Geometry: final body of the model. Coordinates: model frame, mm. A direction names the side the tool comes from. Coordinates: 2 decimals unless noted, no trailing zeros. Write each loop counter-clockwise with the first axis right and the second up, starting at its lowest first coordinate (ties: lowest second). Pieces come first, ordered by that corner, then holes. Notation, with made-up numbers: (6.25, 43) -> (65.25, 43) arc R4 cw to (65.25, 47) -> close; hole circle Ø8 at (33, -2). An arc over 180 degrees is marked (long way). One line per item, written item: value.
```python
from build123d import *

# Parameters (mm, degrees)
BOSS_EXTRUDE1_DEPTH     = 1.5
CUT_EXTRUDE1_DEPTH      = 41.754559874
CUT_EXTRUDE1_DEPTH_BACK = 41.754559874
SKETCH6_R               = 0.5


with BuildPart() as part:
    # Sketch1 → Revolve1 (revolve)
    with BuildSketch(Plane(origin=(-14.777648988, 30.214835565, 34.561537757), x_dir=(-0.025322831104622072, 0, 0.9996793256964189), z_dir=(0.9996793256964189, 0, 0.025322831104622072)), mode=Mode.PRIVATE) as revolve1_sk:
        Polygon((0.538461916, -0.016033073), (-0.794313715, -0.016033073), (-0.794313715, 12.79633963), (-0.794313715, 13.022686392), (0.228391261, 13.022686392), (0.228391261, 12.79633963), (-0.000563715, 12.79633963), (-0.000563715, 11.466008099), (0.538461916, 11.466008099), align=None)
    revolve(revolve1_sk.sketch.rotate(Axis((-14.757534716, 30.388488917, 33.767478758), (0, 1, 0)), 181.451046455), axis=Axis((-14.757534716, 30.388488917, 33.767478758), (0, 1, 0)))

    # Sketch5 → Boss-Extrude1 (add)
    with BuildSketch(Plane(origin=(0, 30.230868638, 0), x_dir=(1, 0, 0), z_dir=(0, 1, 0))):
        Polygon((-14.723785064, -32.435130513), (-14.791284368, -32.435130513), (-14.791284368, -35.099827002), (-14.723785064, -35.099827002), (1.521158766, -35.099827002), (1.521158766, -32.435130513), align=None)
    extrude(amount=BOSS_EXTRUDE1_DEPTH)

    # Sketch6 → Cut-Extrude1 (cut, two sides: drawn at the far end of the back side and taken through both)
    with BuildSketch(Plane.XZ.offset(-30.230868638).offset(-CUT_EXTRUDE1_DEPTH_BACK)):
        with Locations(Location((0.125166735, 33.767478758, 0), (0, 0, 90))):
            Circle(SKETCH6_R)
    extrude(amount=CUT_EXTRUDE1_DEPTH + CUT_EXTRUDE1_DEPTH_BACK, mode=Mode.SUBTRACT)


solid = part.part
```
(1) Pull-direction query (Y, two-part tool) for faces 1 (the flat face through (-15, 30.231, 34)), 2 (the cylindrical face through (-14, 18, 34)), 3 (the flat face through (-7, 31, 32.435)), 4 (the flat face through (-14, 18.749, 33)); classes: released by +Y, released by -Y, zero draft, split by the parting line, or undercut.
Responses:
face 1: released by +Y
face 2: undercut
face 3: zero draft
face 4: undercut
(2) Section C-C (x = -11.5). Return the cut outline in (y, z), then the cut area to 3 significant figures.
Responses:
outline: (30.23, 32.44) -> (31.73, 32.44) -> (31.73, 35.1) -> (30.23, 35.1) -> close
area: 4.00 mm2
(3) Line query: line 1 (Y direction, x = -5.75, z = 34.35); line 2 (X direction, y = 21, z = 32.7); line 3 (X direction, y = 30.75, z = 32.9). Output: solid intervals per line, ascending. Write a range as [from, to].
Responses:
line 1: y = [30.23, 31.73]
line 2: x = [-15.56, -13.96]
line 3: x = [-14.79, 1.52]
(4) Section A-A (z = 33.6). Return the cut outline in (x, y).
Responses:
outline: (-16.08, 18.75) -> (-15.53, 18.75) -> (-15.53, 17.42) -> (-15.77, 17.42) -> (-15.77, 17.19) -> (-13.75, 17.19) -> (-13.75, 17.42) -> (-13.98, 17.42) -> (-13.98, 18.75) -> (-13.44, 18.75) -> (-13.44, 30.23) -> (-0.35, 30.23) -> (-0.35, 31.73) -> (-14.79, 31.73) -> (-14.79, 30.23) -> (-16.08, 30.23) -> close; (0.6, 30.23) -> (1.52, 30.23) -> (1.52, 31.73) -> (0.6, 31.73) -> close
(5) Reachability of faces 5 (the flat face through (-15, 17.192, 34)), 6 (the cylindrical face through (-15.88, 24.57, 33.05)), 7 (the flat face through (-14.791, 31, 34)) from +Z, -Z, +X, -X, +Y, -Y: full face, straight path, thin tool, end or side. Return the list, or none.
Responses:
face 5: +Z, -Z, +X, -X, -Y
face 6: -Y
face 7: +Z, -Z, -X, +Y
(6) Section D-D (y = 23). Return the cut outline in (x, z).
Responses:
outline: circle Ø2.67 at (-14.76, 33.77)
(7) Section B-B (y = 30.75). Return the cut outline in (x, z).
Responses:
outline: (-14.79, 32.44) -> (1.52, 32.44) -> (1.52, 35.1) -> (-14.79, 35.1) -> close; hole circle Ø1 at (0.13, 33.77)
(8) First-contact query: pin 1 (1.5 mm diameter, centred on y = 30, z = 34, fed in from -X); pin 2 (0.8 mm diameter, centred on x = -3.5, z = 33.5, fed in from -Y). Flat tips, straight axial feed; report the tip coordinate or a pass-through.
Responses:
pin 1: stops at x = -16.09
pin 2: stops at y = 30.23
